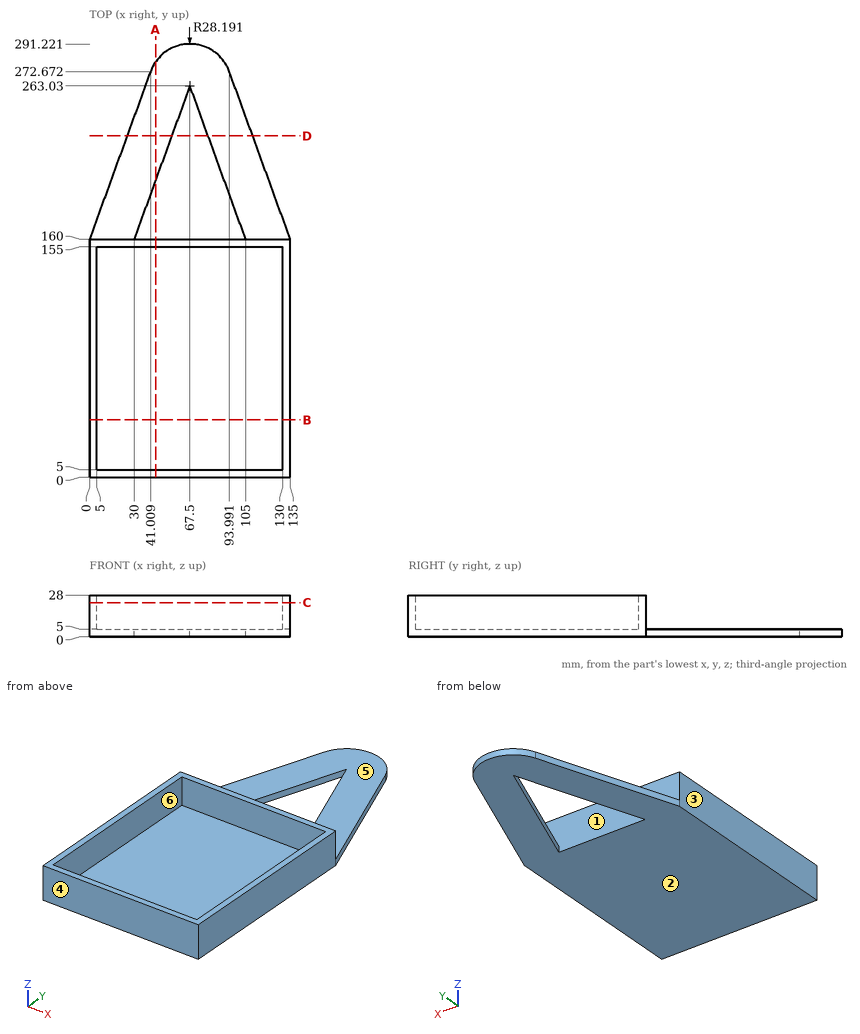
Can you work these out from the drawing? Everything is in mm from the part's minimum corner. A direction names the side the tool comes from. Give positions to 0.01 mm unless a question says otherwise; leave off trailing zeros. Order: outer loops, then holes, each group sorted by start corner. A loop starts at its lowest first (then second) coordinate and runs counter-clockwise, first axis right, second up.
1. Suppose I cut it at A-A (x = 44.5). List the corners of the cut face in (y, z) for me, plus the area to 3 significant figures.
2. We'd pull the mould along X, two halves only. Please class the marked faces 1, 2 and 3: pulls with the +X half, pulls with the -X half, needs draft (parallel to the pull), parting line crosses it, or undercut.
3. I need wall thicknesses on L1, parallel to Y at x = 115, z = 13.25; L2, parallel to X at y = 18.5, z = 10.25; L3, parallel to Z at x = 86, y = 39.5. Which ranges of each line are inside material? Lowest first, please.
4. Will these pins go through, and if not, where does the flat tip stop? P1, Ø5, axis at y = 60.5, z = 21.5, coming from the -X side; P2, Ø1.5, axis at x = 121, y = 198, coming from the +Z side; P3, Ø1.5, axis at x = 96, z = 19, coming from the +Y side.
5. Suppose I cut it at C-C (z = 23). List the corners of the cut face in (x, y) for me, plus the area to 3 significant figures.
6. Suppose I cut it at B-B (y = 38.5). List the corners of the cut face in (x, z) for me.
7. Suppose I cut it at D-D (y = 229.5). List the corners of the cut face in (x, z) for me, plus the area to 3 significant figures.
8. For the marked faces 4, 5 and 6, which set-ups out of +Z, -Z, +X, -X, +Y, -Y let a thin tool reach every point of the face, with its end or its side?
Solved:
1. outline: (0, 0) - (160, 0) - (160, 28) - (155, 28) - (155, 5) - (5, 5) - (5, 28) - (0, 28) - close; (199.84, 0) - (279.33, 0) - (279.33, 5) - (199.84, 5) - close
1. area: 1,430 mm2
2. face 1: undercut
2. face 2: needs draft
2. face 3: pulls with the -X half
3. L1: y = 0 to 5, 155 to 160
3. L2: x = 0 to 5, 130 to 135
3. L3: z = 0 to 5
4. P1: stops at x = 0
4. P2: stops at z = 5
4. P3: stops at y = 160
5. outline: (0, 0) - (135, 0) - (135, 160) - (0, 160) - close; hole (5, 5) - (130, 5) - (130, 155) - (5, 155) - close
5. area: 2,850 mm2
6. outline: (0, 0) - (135, 0) - (135, 28) - (130, 28) - (130, 5) - (5, 5) - (5, 28) - (0, 28) - close
7. outline: (25.3, 0) - (55.3, 0) - (55.3, 5) - (25.3, 5) - close; (79.7, 0) - (109.7, 0) - (109.7, 5) - (79.7, 5) - close
7. area: 300 mm2
8. face 4: +Z, -Z, +X, -X, -Y
8. face 5: +Z, +X, -X, +Y
8. face 6: +Z
